from build123d import *

# Parameters (mm, degrees)
SKETCH1_R           = 22.8
SKETCH1_R_2         = 17
BOSS_EXTRUDE4_DEPTH = 8.8
BOSS_EXTRUDE6_DEPTH = 10
FILLET1_R           = 1.2
FILLET2_R           = 2.4


# Some blends are built 0.0001 mm under size
with BuildPart() as part:
    # Sketch1 → Boss-Extrude4 (new body)
    with BuildSketch(Plane(origin=(0, 0, 0), x_dir=(1, 0, 0), z_dir=(0, 1, 0))):
        with Locations(Location((0, 0, 0), (0, 0, 270))):
            Circle(SKETCH1_R)
        with Locations(Location((0, 0, 0), (0, 0, 270))):
            Circle(SKETCH1_R_2, mode=Mode.SUBTRACT)
    extrude(amount=BOSS_EXTRUDE4_DEPTH)

    # Sketch1<7> → Boss-Extrude6 (add)
    with BuildSketch(Plane(origin=(0, 0, 0), x_dir=(1, 0, 0), z_dir=(0, 1, 0))):
        with BuildLine():
            ThreePointArc((24, 0), (0, 24), (-24, 0))
            Line((-24, 0), (-22.8, 0))
            ThreePointArc((-22.8, 0), (0, 22.8), (22.8, 0))
            Line((22.8, 0), (24, 0))
        make_face()
        with BuildLine():
            Line((-22.8, 0), (-24, 0))
            ThreePointArc((-24, 0), (0, -24), (24, 0))
            Line((24, 0), (22.8, 0))
            ThreePointArc((22.8, 0), (0, -22.8), (-22.8, 0))
        make_face()
    extrude(amount=BOSS_EXTRUDE6_DEPTH)

    # Fillet1
    fillet1_edges = [part.edges().sort_by_distance(p)[0] for p in [
        (-22.8, 8.8, 0),
    ]]
    fillet(fillet1_edges, radius=FILLET1_R - 0.0001)  # a hair under: the kernel refuses the full size

    # Fillet2
    # the kernel refuses this fillet: 2.4 mm, written as the material it takes off along each edge
    with BuildSketch(Plane(origin=(0, 10, 0), x_dir=(1, 0, 0), z_dir=(0, 0, 1))) as fillet2_piece_1:
        with BuildLine():
            CenterArc((21.6, -2.078460969), FILLET2_R, 0, 60)
            Line((24, -2.078460969), (24.048, -2.078460969))
            Line((24.048, -2.078460969), (24.048, 0))
            Line((24.048, 0), (24, 0.048))
            ThreePointArc((24, 0.048), (23.4, 0.048), (22.824, 0.041569219))
            Line((22.824, 0.041569219), (22.8, 0))
        make_face()
    revolve(axis=Axis((0, 10, 0), (0, 1, 0)), mode=Mode.SUBTRACT)


solid = part.part
CAD build for the part. Positions are in the model's coordinates, mm. Round coordinates to 2 decimals unless told otherwise and drop trailing zeros. Write each loop counter-clockwise with the first axis right and the second up, starting at its lowest first coordinate (ties: lowest second). Pieces come first, ordered by that corner, then holes.
(1) Drop flat-ended pins along their axis: P1, Ø1, axis at x = -17.5, z = -10, coming from the +Y side; P2, Ø5, axis at y = 2, z = 7, coming from the +X side; P3, Ø6, axis at y = 6.5, z = 10, coming from the -X side; P4, Ø12, axis at x = -3.5, z = -8.5, coming from the -Y side. Give the stop position or say it passes through.
(2) Slice it at C-C, the plane y = 2.5. Write the cut outline in (x, z).
(3) Mould opens along Z. For faces 1 (the face through (-22.89, 3.91, 7.21)), 2 (the face through (-5.7, 0, -16.3)), 3 (the face through (16.855, 4.338, -2.213)) say: pulls with the +Z half, pulls with the -Z half, needs draft (parallel to the pull), parting line crosses it, or undercut.
(4) Probe line 1 along X through (y, z) = (6.5, 0); line 2 along X through (y, z) = (3.5, -4.5); line 3 along Z through (x, y) = (11.5, 5.5). List the from-to ranges inside material, lowest first.
From the geometry:
1. P1: stops at y = 8.8
1. P2: stops at x = 23.57
1. P3: stops at x = -22.96
1. P4: passes through
2. outline: circle Ø48 at (0, 0); hole circle Ø34 at (0, 0)
3. face 1: parting line crosses it
3. face 2: needs draft
3. face 3: undercut
4. line 1: x = -24 to -17, 17 to 24
4. line 2: x = -23.57 to -16.39, 16.39 to 23.57
4. line 3: z = -21.07 to -12.52, 12.52 to 21.07
